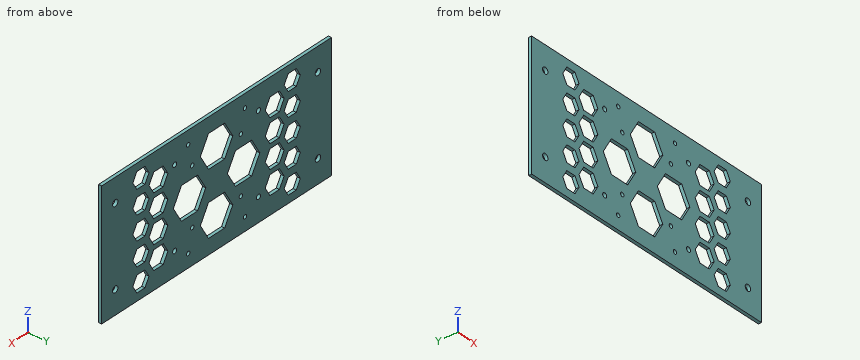
```python
from build123d import *

# Parameters (mm, degrees)
SKETCH_1_W          = 170
SKETCH_1_H          = 80
SKETCH_1_R          = 2
SKETCH_1_R_2        = 1.25
SKETCH_1_R_3        = 1.5
EXTRUDE_1_DEPTH     = 2
CUT_EXTRUDE_1_DEPTH = 50
CUT_EXTRUDE_2_DEPTH = 50
CUT_EXTRUDE_3_DEPTH = 50


with BuildPart() as part:
    # 草图1 → 凸台-拉伸1 (new body)
    with BuildSketch(Plane(origin=(0, 0, 0), x_dir=(1, 0, 0), z_dir=(0, 1, 0))):
        with Locations((85, 40)):
            Rectangle(SKETCH_1_W, SKETCH_1_H)
        with Locations(Location((10, 65, 0), (0, 0, 270))):
            Circle(SKETCH_1_R, mode=Mode.SUBTRACT)
        with Locations(Location((10, 15, 0), (0, 0, 90))):
            Circle(SKETCH_1_R, mode=Mode.SUBTRACT)
        with Locations(Location((160, 15, 0), (0, 0, 270))):
            Circle(SKETCH_1_R, mode=Mode.SUBTRACT)
        with Locations(Location((160, 65, 0), (0, 0, 90))):
            Circle(SKETCH_1_R, mode=Mode.SUBTRACT)
        with Locations(Location((67, 58, 0), (0, 0, 270))):
            Circle(SKETCH_1_R_2, mode=Mode.SUBTRACT)
        with Locations(Location((67, 22, 0), (0, 0, 90))):
            Circle(SKETCH_1_R_2, mode=Mode.SUBTRACT)
        with Locations(Location((103, 22, 0), (0, 0, 270))):
            Circle(SKETCH_1_R_2, mode=Mode.SUBTRACT)
        with Locations(Location((103, 58, 0), (0, 0, 90))):
            Circle(SKETCH_1_R_2, mode=Mode.SUBTRACT)
        with Locations(Location((64, 71.5, 0), (0, 0, 270))):
            Circle(SKETCH_1_R_2, mode=Mode.SUBTRACT)
        with Locations(Location((64, 8.5, 0), (0, 0, 90))):
            Circle(SKETCH_1_R_2, mode=Mode.SUBTRACT)
        with Locations(Location((106, 8.5, 0), (0, 0, 270))):
            Circle(SKETCH_1_R_2, mode=Mode.SUBTRACT)
        with Locations(Location((106, 71.5, 0), (0, 0, 90))):
            Circle(SKETCH_1_R_2, mode=Mode.SUBTRACT)
        with Locations(Location((54, 65, 0), (0, 0, 270))):
            Circle(SKETCH_1_R_3, mode=Mode.SUBTRACT)
        with Locations(Location((54, 15, 0), (0, 0, 90))):
            Circle(SKETCH_1_R_3, mode=Mode.SUBTRACT)
        with Locations(Location((116, 15, 0), (0, 0, 270))):
            Circle(SKETCH_1_R_3, mode=Mode.SUBTRACT)
        with Locations(Location((116, 65, 0), (0, 0, 90))):
            Circle(SKETCH_1_R_3, mode=Mode.SUBTRACT)
    extrude(amount=EXTRUDE_1_DEPTH)

    # 草图3 → 切除-拉伸1 (cut)
    with BuildSketch(Plane(origin=(0, 2, 0), x_dir=(1, 0, 0), z_dir=(0, 1, 0))):
        Polygon((26, 15.173938425), (23, 9.977786002), (26, 4.781633579), (32, 4.781633579), (35, 9.977786002), (32, 15.173938425), align=None)
        Polygon((38.5, 23.545517328), (35, 17.483339502), (38.5, 11.421161675), (45.5, 11.421161675), (49, 17.483339502), (45.5, 23.545517328), align=None)
        Polygon((32, 30.185045424), (26, 30.185045424), (23, 24.988893001), (26, 19.792740578), (32, 19.792740578), (35, 24.988893001), align=None)
        Polygon((45.5, 38.556624327), (38.5, 38.556624327), (35, 32.494446501), (38.5, 26.432268674), (45.5, 26.432268674), (49, 32.494446501), align=None)
        Polygon((32, 45.196152423), (26, 45.196152423), (23, 40), (26, 34.803847577), (32, 34.803847577), (35, 40), align=None)
        Polygon((49, 47.505553499), (45.5, 41.443375673), (38.5, 41.443375673), (35, 47.505553499), (38.5, 53.567731326), (45.5, 53.567731326), align=None)
        Polygon((45.5, 56.454482672), (38.5, 56.454482672), (35, 62.516660498), (38.5, 68.578838325), (45.5, 68.578838325), (49, 62.516660498), align=None)
        Polygon((35, 55.011106999), (32, 49.814954576), (26, 49.814954576), (23, 55.011106999), (26, 60.207259422), (32, 60.207259422), align=None)
        Polygon((32, 64.826061575), (26, 64.826061575), (23, 70.022213998), (26, 75.218366421), (32, 75.218366421), (35, 70.022213998), align=None)
        Polygon((144, 64.826061575), (147, 70.022213998), (144, 75.218366421), (138, 75.218366421), (135, 70.022213998), (138, 64.826061575), align=None)
        Polygon((138, 49.814954576), (144, 49.814954576), (147, 55.011106999), (144, 60.207259422), (138, 60.207259422), (135, 55.011106999), align=None)
        Polygon((131.5, 56.454482672), (135, 62.516660498), (131.5, 68.578838325), (124.5, 68.578838325), (121, 62.516660498), (124.5, 56.454482672), align=None)
        Polygon((124.5, 41.443375673), (131.5, 41.443375673), (135, 47.505553499), (131.5, 53.567731326), (124.5, 53.567731326), (121, 47.505553499), align=None)
        Polygon((135, 40), (138, 45.196152423), (144, 45.196152423), (147, 40), (144, 34.803847577), (138, 34.803847577), align=None)
        Polygon((121, 32.494446501), (124.5, 38.556624327), (131.5, 38.556624327), (135, 32.494446501), (131.5, 26.432268674), (124.5, 26.432268674), align=None)
        Polygon((135, 24.988893001), (138, 30.185045424), (144, 30.185045424), (147, 24.988893001), (144, 19.792740578), (138, 19.792740578), align=None)
        Polygon((124.5, 23.545517328), (131.5, 23.545517328), (135, 17.483339502), (131.5, 11.421161675), (124.5, 11.421161675), (121, 17.483339502), align=None)
        Polygon((138, 15.173938425), (144, 15.173938425), (147, 9.977786002), (144, 4.781633579), (138, 4.781633579), (135, 9.977786002), align=None)
    extrude(amount=-CUT_EXTRUDE_1_DEPTH, mode=Mode.SUBTRACT)

    # 草图4 → 切除-拉伸2 (cut)
    with BuildSketch(Plane(origin=(0, 2, 0), x_dir=(1, 0, 0), z_dir=(0, 1, 0))):
        Polygon((77, 40), (71, 50.392304845), (59, 50.392304845), (53, 40), (59, 29.607695155), (71, 29.607695155), align=None)
        Polygon((99, 29.607695155), (93, 40), (99, 50.392304845), (111, 50.392304845), (117, 40), (111, 29.607695155), align=None)
    extrude(amount=-CUT_EXTRUDE_2_DEPTH, mode=Mode.SUBTRACT)

    # 草图5 → 切除-拉伸3 (cut)
    with BuildSketch(Plane(origin=(0, 2, 0), x_dir=(1, 0, 0), z_dir=(0, 1, 0))):
        Polygon((91, 30.392304845), (79, 30.392304845), (73, 20), (79, 9.607695155), (91, 9.607695155), (97, 20), align=None)
        Polygon((97, 60), (91, 49.607695155), (79, 49.607695155), (73, 60), (79, 70.392304845), (91, 70.392304845), align=None)
    extrude(amount=-CUT_EXTRUDE_3_DEPTH, mode=Mode.SUBTRACT)


solid = part.part
```
Can you work these out from the model? Positions are in its coordinate system, mm. Round coordinates to 2 decimals unless told otherwise and drop trailing zeros. Order: outer loops, then holes, each group sorted by start corner. A loop starts at its lowest first (then second) coordinate and runs counter-clockwise, first axis right, second up. Notation, with made-up numbers: (-36, -5.5) -> (23, -5.5) arc R19 cw to (23, -1.5) -> close; hole circle Ø2 at (-35.5, 34). An arc over 180 degrees is marked (long way). Return JSON: item names as keys, results as strings. Group by question number.
1. If we section it at B-B, the plane x = 142: Write out the boundary of the cut face in (y, z), then the cut area to 3 significant figures.
2. If we section it at A-A, the plane x = 10: Write out the boundary of the cut face in (y, z).
3. I need wall thicknesses on line 1 (Z direction, x = 67, y = 0.85); line 2 (Z direction, x = 42, y = 1.1); line 3 (X direction, y = 1.75, z = -31). Which ranges of each line are inside material? Lowest first, please. Write a range as [from, to].
4. If we section it at C-C, the plane y = 1.7: Count the separate pieces of the cut face and the enclosed holes in it, then the cut area to 3 significant figures.
Output values:
{
 "1": {"outline": "(0, -80) -> (2, -80) -> (2, -75.22) -> (0, -75.22) -> close; (0, -64.83) -> (2, -64.83) -> (2, -60.21) -> (0, -60.21) -> close; (0, -49.81) -> (2, -49.81) -> (2, -45.2) -> (0, -45.2) -> close; (0, -34.8) -> (2, -34.8) -> (2, -30.19) -> (0, -30.19) -> close; (0, -19.79) -> (2, -19.79) -> (2, -15.17) -> (0, -15.17) -> close; (0, -4.78) -> (2, -4.78) -> (2, 0) -> (0, 0) -> close", "area": "56.1 mm²"},
 "2": {"outline": "(0, -80) -> (2, -80) -> (2, -67) -> (0, -67) -> close; (0, -63) -> (2, -63) -> (2, -17) -> (0, -17) -> close; (0, -13) -> (2, -13) -> (2, 0) -> (0, 0) -> close"},
 "3": {"line 1": "[-80, -59.25], [-56.75, -50.39], [-29.61, -23.25], [-20.75, 0]", "line 2": "[-80, -68.58], [-56.45, -53.57], [-41.44, -38.56], [-26.43, -23.55], [-11.42, 0]", "line 3": "[0, 35.86], [48.14, 58.2], [71.8, 98.2], [111.8, 121.86], [134.14, 170]"},
 "4": {"separate pieces": "1", "enclosed holes": "38", "area": "10,000 mm²"}
}
